Design review of the part built by this model. Coordinates are the model's own, in mm. Face numbers are marked on the shaded views. A direction names the side the tool comes from. Give positions to 0.01 mm unless a question says otherwise; leave off trailing zeros. Loops run counter-clockwise (first coordinate to the right, second up) from the corner with the lowest first, then second, coordinate; pieces in that order, holes last.
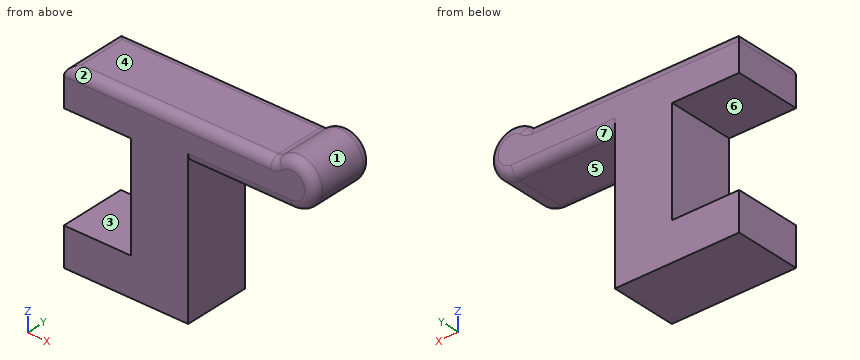
from build123d import *

# Parameters (mm, degrees)
F1_DEPTH = 35
F2_F1_R  = 5
F2_F2_R  = 5


with BuildPart() as f1:
    # F0 (on Front) → F1 (new body)
    with BuildSketch(Plane.XZ):
        with BuildLine():
            Line((0, 20), (0, 0))
            Line((0, 0), (65, 0))
            Line((65, 0), (65, 75))
            Line((65, 75), (118.94427191, 75))
            ThreePointArc((118.94427191, 75), (129.8987230601, 91.8989794856), (110, 95))
            Line((110, 95), (0, 95))
            Line((0, 95), (0, 75))
            Line((0, 75), (35, 75))
            Line((35, 75), (35, 20))
            Line((35, 20), (0, 20))
        make_face()
    extrude(amount=F1_DEPTH)

    # F2: fillet of radius 5 on 4 edges, made by hand

    # F2_f1
    f2_f1_edges = [f1.edges().sort_by_distance(p)[0] for p in [
        (110, -17.5, 95),
    ]]
    fillet(f2_f1_edges, radius=F2_F1_R)

    # F2_f2
    f2_f2_edges = [f1.edges().sort_by_distance(p)[0] for p in [
        (0, -17.5, 95),
        (53.9949103799, 0, 95),
        (53.9949103799, -35, 95),
        (109.7048066113, -35, 95.3033178169),
        (109.7048066113, 0, 95.3033178169),
    ]]
    fillet(f2_f2_edges, radius=F2_F2_R)


solid = f1.part
Q1. Draft analysis for pull direction Z (two halves, no side actions). For the marked faces 1, 2 and 3, state which applies: pulls with the +Z half, pulls with the -Z half, needs draft (parallel to the pull), parting line crosses it, or undercut.
Results:
face 1: parting line crosses it
face 2: pulls with the +Z half
face 3: undercut
Q2. Take a section at A-A (y = -10). Give the boundary of the cut face in (x, z).
Results:
outline: (0, 0) - (65, 0) - (65, 75) - (118.94, 75) arc R12 ccw (long way) to (111.21, 96.18) arc R5 cw to (107.99, 95) - (5, 95) arc R5 ccw to (0, 90) - (0, 75) - (35, 75) - (35, 20) - (0, 20) - close
Q3. Take a section at C-C (z = 55). Give the boundary of the cut face in (x, y), plus the area to 3 significant figures.
Results:
outline: (35, -35) - (65, -35) - (65, 0) - (35, 0) - close
area: 1,050 mm2
Q4. Tool access review of the marked faces 4, 5, 6 and 7: name each direction out of +Z, -Z, +X, -X, +Y, -Y from which nothing blocks a thin tool from reaching the whole face with its end or side.
Results:
face 4: +Z, -X, +Y, -Y
face 5: -Z, +X, +Y, -Y
face 6: -X, +Y, -Y
face 7: -Z, +X, +Y
Q5. Wall thickness on line 1 (Z direction, x = 30, y = -17); line 2 (X direction, y = -31, z = 13); line 3 (X direction, y = -15.5, z = 63): over which ranges is each line inside the solid? List them lowest first.
Results:
line 1: z = 0 to 20, 75 to 95
line 2: x = 0 to 65
line 3: x = 35 to 65
Q6. Insertion check: pin 1 (1.5 mm diameter, centred on x = 106.5, z = 75, fed in from -Y); pin 2 (3 mm diameter, centred on x = 17, y = -5.5, fed in from -Z); pin 3 (10.5 mm diameter, centred on y = -9, z = 40, fed in from -X); pin 4 (2 mm diameter, centred on x = 81, y = -3.5, fed in from +Z). Each pin has a flat end and moves straight along its axis. Give the tip position at first contact, or say it passes through.
Results:
pin 1: stops at y = -32.63
pin 2: stops at z = 0
pin 3: stops at x = 35
pin 4: stops at z = 94.97
Q7. Take a section at D-D (x = 50.5). Give the boundary of the cut face in (y, z), plus the area to 3 significant figures.
Results:
outline: (-35, 0) - (0, 0) - (0, 90) arc R5 ccw to (-5, 95) - (-30, 95) arc R5 ccw to (-35, 90) - close
area: 3,310 mm2
Q8. Take a section at B-B (x = 73). Give the boundary of the cut face in (y, z), plus the area to 3 significant figures.
Results:
outline: (-35, 80) arc R5 ccw to (-30, 75) - (-5, 75) arc R5 ccw to (0, 80) - (0, 90) arc R5 ccw to (-5, 95) - (-30, 95) arc R5 ccw to (-35, 90) - close
area: 679 mm2
